Source: CAD feature listing. Evaluate the final solid. Frame: model axes, mm. Face numbers are marked on the shaded views. A direction names the side the tool comes from. Round coordinates to 2 decimals unless told otherwise and drop trailing zeros. Write each loop counter-clockwise with the first axis right and the second up, starting at its lowest first coordinate (ties: lowest second). Pieces come first, ordered by that corner, then holes. Notation, with made-up numbers: (39, 67.25) -> (43, 67.25) arc R27 cw to (43, 92.25) -> close; hole circle Ø2 at (55.5, 30.25). An arc over 180 degrees is marked (long way). Return JSON: item names as keys, results as strings. Group by question number.
Autodesk Inventor part; units mm, degrees
ref_plane "YZ Plane" through (0, 0, 0) normal (1, 0, 0) x (0, 1, 0)
ref_plane "XZ Plane" through (0, 0, 0) normal (0, 1, 0) x (-1, 0, 0)
ref_plane "XY Plane" through (0, 0, 0) normal (0, 0, 1) x (1, 0, 0)
sketch "스케치1" plane through (0, 0, 0) normal (0, 1, 0) x (-1, 0, 0)
  line L0 (124.1226, 0) -> (-124.1226, 0)
  line L1 (0, -98.3487) -> (0, 29.2174)
  line L2 (63.5, 0) -> (-63.5, 0)
  arc A0 (88.5, -4) -> (63.5, 0) centre (63.5, -80.125) ccw
  line L3 (63.5, 0) -> (63.5, 10)
  line L4 (88.5, -4) -> (88.5, 6)
  arc A1 (88.5, 6) -> (63.5, 10) centre (63.5, -70.125) ccw
  line L5 (63.5, 10) -> (0, 10)
  arc A2 (-63.5, 0) -> (-88.5, -4) centre (-63.5, -80.125) ccw
  line L6 (-63.5, 0) -> (-63.5, 10)
  line L7 (-88.5, -4) -> (-88.5, 6)
  arc A3 (-63.5, 10) -> (-88.5, 6) centre (-63.5, -70.125) ccw
  point P0 (0, 0)
  dimension "d0" = 127
  dimension "d1" = 10
  dimension "d2" = 10
  dimension "d3" = 14
  dimension "d4" = 25
extrude "돌출1" add sketch "스케치1" along normal blind 20 contours L4 A0 L0 | A2 L7 L0 | L0 L7 A3 L6 | L0 L3 A1 L4
sketch "스케치2" plane through (0, 20, 0) normal (0, 1, 0) x (1, 0, 0)
  point P0 (0, 0)
sketch "스케치3" plane through (0, 20, 0) normal (0, 1, 0) x (1, 0, 0)
  line L0 (-63.5, -10) -> (-63.5, 0)
  arc A0 (-88.5, 4) -> (-63.5, 0) centre (-63.5, 80.125) ccw
  line L1 (-88.5, 4) -> (-88.5, -6)
  arc A1 (-88.5, -6) -> (-63.5, -10) centre (-63.5, 70.125) ccw
  line L2 (88.5, -6) -> (88.5, 4)
  arc A2 (63.5, 0) -> (88.5, 4) centre (63.5, 80.125) ccw
  line L3 (63.5, 0) -> (63.5, -10)
  arc A3 (63.5, -10) -> (88.5, -6) centre (63.5, 70.125) ccw
  line L4 (-63.5, -10) -> (63.5, -10)
  line L5 (63.5, -10) -> (63.5, 0)
  line L6 (63.5, 0) -> (-63.5, 0)
  line L7 (-63.5, 0) -> (-63.5, -10)
  line L8 (-88.5, 4) -> (88.5, 4)
  point P0 (0, 0)
extrude "돌출2" add sketch "스케치3" along normal blind 20
sketch "스케치4" plane through (0, 0, 0) normal (1, 0, 0) x (0, 1, 0)
  line L0 (40, 10) -> (32.2354, 38.9778)
  line L1 (40, 6) -> (40, 10)
  line L2 (40, -4) -> (60, -4)
  line L3 (32.2354, 38.9778) -> (45, 38.9778)
  line L4 (40, 6) -> (40, -4)
  line L5 (45, 38.9778) -> (45, 11)
  line L6 (60, 11) -> (60, -4)
  line L7 (0, 6) -> (40, 6)
  line L8 (60, 11) -> (45, 11)
  point P0 (0, 0)
  point P1 (20, 10)
  dimension "d9" = 165
  dimension "d11" = 30
  dimension "d12" = 20
  dimension "d13" = 5
  dimension "d16" = 15
extrude "돌출3" add sketch "스케치4" along normal mid plane 40
sketch "스케치5" plane through (88.5, 20, -4) normal (0, 0, -1) x (-1, 0, 0)
  line L0 (0, 0) -> (177, 0)
  line L1 (177, 0) -> (177, 20)
  line L2 (108.5, 20) -> (177, 20)
  line L3 (108.5, 40) -> (108.5, 20)
  line L4 (108.5, 40) -> (68.5, 40)
  line L5 (68.5, 20) -> (68.5, 40)
  line L6 (0, 20) -> (68.5, 20)
  line L7 (0, 0) -> (0, 20)
  line L8 (68.5, 30) -> (108.5, 30)
  circle A0 centre (78.5056, 30) radius 2
  circle A1 centre (98.5056, 30) radius 2
  point P0 (88.5, -20)
  dimension "d17" = 4
  dimension "d18" = 4
  dimension "d19" = 20
extrude "돌출4" cut sketch "스케치5" against normal blind 40 contours A0 L8 | L8 A0 | A1 L8 | L8 A1
sketch "스케치6" plane through (88.5, 20, -4) normal (0, 0, -1) x (-1, 0, 0)
  circle A0 centre (78.5056, 30) radius 2
  circle A1 centre (98.5056, 30) radius 2
  circle A2 centre (78.5056, 30) radius 4
  circle A3 centre (98.5056, 30) radius 4
  point P0 (88.5, -20)
  dimension "d22" = 8
  dimension "d23" = 8
extrude "돌출5" cut sketch "스케치6" against normal blind 4 contours A0 | A2 | A3
properties part number "라이다 고정"
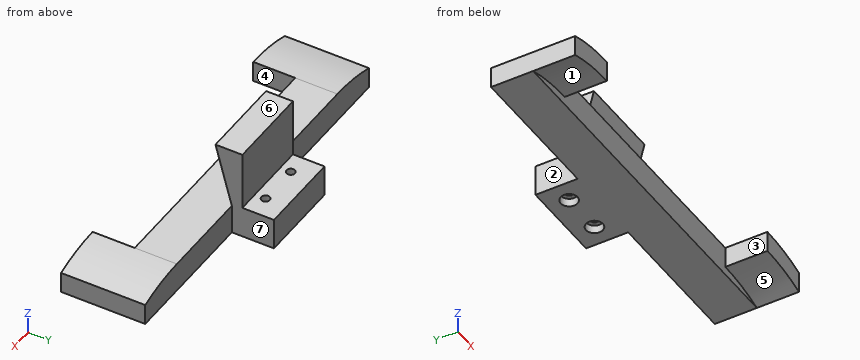
Item 1: Cut plane D-D on y = 42. Output: boundary loops of the cut face in (x, z).
Item 2: Material intervals for probe 1 along Y at (x, z) = (10, 7); probe 2 along Z at (x, y) = (-48, 23); probe 3 along X at (y, z) = (9, 2), sorted ascending.
Item 3: Cut plane A-A on y = 50. Output: boundary loops of the cut face in (x, z), and give its area (3 significant figures).
Item 4: Cut plane B-B on z = 8. Output: boundary loops of the cut face in (x, y).
Item 5: First-contact query: pin 1 Ø11 at (x, z) = (-41, 2.5) entering from +Y; pin 2 Ø6.5 at (x, y) = (9.99, 50) entering from +Z; pin 3 Ø8.5 at (y, z) = (43.5, 26.5) entering from +X. Flat tips, straight axial feed; report the tip coordinate or a pass-through.
Item 6: Pull-direction query (X, two-part tool) for the marked faces 4, 5, 6 and 7; classes: +X half, -X half, draft (parallel to the pull), parting line (faces both ways), or undercut.
Item 7: Set-up query: the marked faces 1, 2 and 3. Return all of +Z, -Z, +X, -X, +Y, -Y with unobstructed straight access to the full face (end or side cutting, diameter ignored); none if empty.
Item 8: Cut plane C-C on x = -61. Output: boundary loops of the cut face in (y, z), and give its area (3 significant figures).
Here are the results:
{
 "1": {"outline": "(-20, -4) -> (20, -4) -> (20, 38.98) -> (-20, 38.98) -> close"},
 "2": {"probe 1": "y = 20 to 48, 52 to 60", "probe 2": "z = -4 to 10", "probe 3": "x = -88.5 to -63.5, 63.5 to 88.5"},
 "3": {"outline": "(-20, -4) -> (-14.01, -4) -> (-14.01, 0) -> (-12.01, 0) -> (-12.01, 11) -> (-20, 11) -> close; (-8.01, 0) -> (-6.01, 0) -> (-6.01, -4) -> (5.99, -4) -> (5.99, 0) -> (7.99, 0) -> (7.99, 11) -> (-8.01, 11) -> close; (11.99, 0) -> (13.99, 0) -> (13.99, -4) -> (20, -4) -> (20, 11) -> (11.99, 11) -> close", "area": "448 mm^2"},
 "4": {"outline": "(-81.29, 0) -> (-63.5, 0) -> (-63.5, 20) -> (63.5, 20) -> (63.5, 0) -> (81.29, 0) -> (81.29, 40) -> (20, 40) -> (20, 60) -> (-20, 60) -> (-20, 40) -> (-81.29, 40) -> close; hole circle Ø4 at (-10.01, 50); hole circle Ø4 at (9.99, 50)"},
 "5": {"pin 1": "stops at y = 40", "pin 2": "stops at z = 11", "pin 3": "stops at x = 20"},
 "6": {"face 4": "undercut", "face 5": "undercut", "face 6": "draft", "face 7": "+X half"},
 "7": {"face 1": "-Z, -Y", "face 2": "+Z, -X, +Y", "face 3": "+Z, -Z, -Y"},
 "8": {"outline": "(20, -4) -> (40, -4) -> (40, 10) -> (20, 10) -> close", "area": "280 mm^2"}
}
